```python
from build123d import *

# Parameters (mm, degrees)
SKETCH1_W           = 60
SKETCH1_H           = 40
BOSS_EXTRUDE1_DEPTH = 5
SKETCH4_R           = 2.25
CUT_EXTRUDE2_DEPTH  = 37.400549446
SKETCH6_R           = 10.5
SKETCH6_R_2         = 2
CUT_EXTRUDE3_DEPTH  = 37.400549446


with BuildPart() as part:
    # Sketch1 → Boss-Extrude1 (new body)
    with BuildSketch(Plane(origin=(0, 0, 0), x_dir=(1, 0, 0), z_dir=(0, 1, 0))):
        Rectangle(SKETCH1_W, SKETCH1_H)
    extrude(amount=BOSS_EXTRUDE1_DEPTH)

    # Sketch4 → Cut-Extrude2 (cut, through all)
    with BuildSketch(Plane(origin=(0, 5, 0), x_dir=(1, 0, 0), z_dir=(0, 1, 0))):
        with Locations(Location((20, 12, 0), (0, 0, 270))):
            Circle(SKETCH4_R)
        with Locations(Location((20, -12, 0), (0, 0, 90))):
            Circle(SKETCH4_R)
    extrude(amount=-CUT_EXTRUDE2_DEPTH, mode=Mode.SUBTRACT)

    # Sketch6 → Cut-Extrude3 (cut, through all)
    with BuildSketch(Plane(origin=(0, 5, 0), x_dir=(1, 0, 0), z_dir=(0, 1, 0))):
        with Locations(Location((-10.000056756, -7.4323e-05, 0), (0, 0, 270))):
            Circle(SKETCH6_R)
        with Locations(Location((-20.606658473, 10.606527395, 0), (0, 0, 270))):
            Circle(SKETCH6_R_2)
        with Locations(Location((0.606544962, 10.606527395, 0), (0, 0, 270))):
            Circle(SKETCH6_R_2)
        with Locations(Location((0.606544962, -10.606676041, 0), (0, 0, 270))):
            Circle(SKETCH6_R_2)
        with Locations(Location((-20.606658473, -10.606676041, 0), (0, 0, 270))):
            Circle(SKETCH6_R_2)
    extrude(amount=-CUT_EXTRUDE3_DEPTH, mode=Mode.SUBTRACT)


solid = part.part
```
Input: part model. Units: mm. Frame: model coordinates. Round coordinates to 2 decimals unless told otherwise and drop trailing zeros. Loops run counter-clockwise (first coordinate to the right, second up) from the corner with the lowest first, then second, coordinate; pieces in that order, holes last. Notation, with made-up numbers: (76, -2) -> (110, -2) arc R29 cw to (110, 20) -> close; hole circle Ø7 at (-11, -13). An arc over 180 degrees is marked (long way). One line per item, written item: value.
(1) Section B-B (y = 2.7). Return the cut outline in (x, z), plus the area to 3 significant figures.
Geometry check:
outline: (-30, -20) -> (30, -20) -> (30, 20) -> (-30, 20) -> close; hole circle Ø4 at (-20.61, -10.61); hole circle Ø4 at (-20.61, 10.61); hole circle Ø21 at (-10, 0); hole circle Ø4 at (0.61, -10.61); hole circle Ø4 at (0.61, 10.61); hole circle Ø4.5 at (20, -12); hole circle Ø4.5 at (20, 12)
area: 1,970 mm2
(2) Pin query (flat end, axial travel): pin 1 (1.5 mm diameter, centred on x = -9.5, z = 10, fed in from -Y). Return the tip coordinate at first contact, or that it passes through.
Geometry check:
pin 1: y = 0
(3) Mould query, pull axis Z, two halves, no side actions, for faces 1 (the face through (0, 2, 20)), 2 (the face through (0, 2, -20)), 3 (the face through (22.196, 2.535, 12.488)), 4 (the face through (30, 2, 0)). Classes: pulls with the +Z half, pulls with the -Z half, needs draft (parallel to the pull), parting line crosses it, or undercut.
Geometry check:
face 1: pulls with the +Z half
face 2: pulls with the -Z half
face 3: undercut
face 4: needs draft
(4) Section D-D (z = -12). Return the cut outline in (x, y), plus the area to 3 significant figures.
Geometry check:
outline: (-30, 0) -> (-22.04, 0) -> (-22.04, 5) -> (-30, 5) -> close; (-19.17, 0) -> (-0.83, 0) -> (-0.83, 5) -> (-19.17, 5) -> close; (2.04, 0) -> (17.75, 0) -> (17.75, 5) -> (2.04, 5) -> close; (22.25, 0) -> (30, 0) -> (30, 5) -> (22.25, 5) -> close
area: 249 mm2
(5) Section A-A (x = 20). Return the cut outline in (y, z), plus the area to 3 significant figures.
Geometry check:
outline: (0, -20) -> (5, -20) -> (5, -14.25) -> (0, -14.25) -> close; (0, -9.75) -> (5, -9.75) -> (5, 9.75) -> (0, 9.75) -> close; (0, 14.25) -> (5, 14.25) -> (5, 20) -> (0, 20) -> close
area: 155 mm2
(6) Material intervals for line 1 (X direction, y = 2.3, z = -0.5); line 2 (X direction, y = 2.2, z = -12); line 3 (Z direction, x = 21.5, y = 4.2), sorted ascending. Write a range as [from, to].
Geometry check:
line 1: [-30, -20.49], [0.49, 30]
line 2: [-30, -22.04], [-19.17, -0.83], [2.04, 17.75], [22.25, 30]
line 3: [-20, -13.68], [-10.32, 10.32], [13.68, 20]
(7) Section C-C (z = 7). Return the cut outline in (x, y), plus the area to 3 significant figures.
Geometry check:
outline: (-30, 0) -> (-17.83, 0) -> (-17.83, 5) -> (-30, 5) -> close; (-2.17, 0) -> (30, 0) -> (30, 5) -> (-2.17, 5) -> close
area: 222 mm2
